Input: part model. Units: mm. Frame: model coordinates. Face numbers are marked on the shaded views. A direction names the side the tool comes from. Give positions to 0.01 mm unless a question says otherwise; leave off trailing zeros. Loops run counter-clockwise (first coordinate to the right, second up) from the corner with the lowest first, then second, coordinate; pieces in that order, holes last.
from build123d import *

# Parameters (mm, degrees)
F0_W     = 31.75
F0_H     = 82.55
F1_DEPTH = 6.35
F3_DEPTH = 6.35
F2_W     = 12.7
F2_H     = 29.119744
F4_DEPTH = 31.75
F6_DEPTH = 44.45
F8_DEPTH = 6.35


with BuildPart() as f1:
    # F0 (on Top) → F1 (new body)
    with BuildSketch(Plane.XY):
        with Locations((15.875, 0)):
            Rectangle(F0_W, F0_H)
    extrude(amount=F1_DEPTH)

    # F2 (on face) → F3 (join)
    with BuildSketch(Plane.YZ.offset(31.75)):
        Polygon((-41.275, 44.45), (-41.275, 6.35), (31.205256, 6.35), (-19.594744, 44.45), (-19.594744, 53.430256), (-32.294744, 53.430256), align=None)
        with BuildLine():
            ThreePointArc((-12.355744, 28.448), (-10.704744, 27.305), (-10.069744, 25.4))
            ThreePointArc((-10.069744, 25.4), (-10.704744, 23.495), (-12.355744, 22.352))
            ThreePointArc((-12.355744, 22.352), (-13.244744, 22.225), (-14.133744, 22.352))
            ThreePointArc((-14.133744, 22.352), (-16.419744, 25.4), (-14.133744, 28.448))
            ThreePointArc((-14.133744, 28.448), (-13.244744, 28.575), (-12.355744, 28.448))
        make_face(mode=Mode.SUBTRACT)
        with BuildLine():
            Line((-12.355744, 22.352), (-12.355744, 28.448))
            ThreePointArc((-12.355744, 28.448), (-13.244744, 28.575), (-14.133744, 28.448))
            Line((-14.133744, 28.448), (-14.133744, 22.352))
            ThreePointArc((-14.133744, 22.352), (-13.244744, 22.225), (-12.355744, 22.352))
        make_face()
    extrude(amount=-F3_DEPTH)

    # F2 (on face) → F4 (join)
    with BuildSketch(Plane.YZ.offset(31.75)):
        with Locations((-25.944744, 67.990128)):
            Rectangle(F2_W, F2_H)
    extrude(amount=-F4_DEPTH)

    # F5 (on face) → F6 (join)
    with BuildSketch(Plane.XZ.offset(41.275)):
        Polygon((25.4, 6.35), (0, 6.35), (0, 0), (31.75, 0), (31.75, 6.35), align=None)
    extrude(amount=F6_DEPTH)

    # F7 (on face) → F8 (join)
    with BuildSketch(Plane.YZ.offset(31.75)):
        Polygon((-41.275, 44.45), (-85.725, 6.35), (-79.375, 6.35), (-41.275, 39.007143), align=None)
    extrude(amount=-F8_DEPTH)

    # F9: F1 across plane


with BuildPart() as f1_1:
    add(f1.part)
    add(f1.part.mirror(Plane.YZ))


solid = f1_1.part
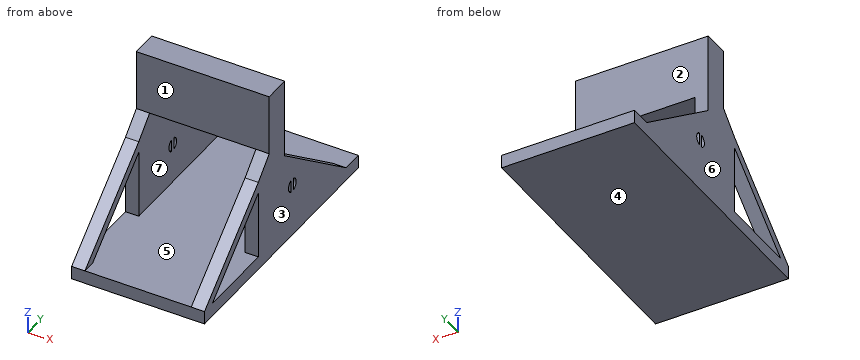
(1) Pin query (flat end, axial travel): pin 1 Ø3 at (x, z) = (29.5, 26) entering from +Y; pin 2 Ø5 at (x, z) = (-29.5, 31) entering from -Y; pin 3 Ø3 at (x, y) = (20.5, -16.5) entering from -Z; pin 4 Ø23.5 at (x, z) = (10, 69.5) entering from -Y. Return the tip coordinate at first contact, or that it passes through.
Values follow:
pin 1: stops at y = 7.01
pin 2: stops at y = -59.88
pin 3: stops at z = 0
pin 4: stops at y = -32.29
(2) Mould query, pull axis X, two halves, no side actions, for the marked faces 4, 5, 6 and 7. Classes: +X half, -X half, draft (parallel to the pull), parting line (faces both ways), or undercut.
Values follow:
face 4: draft
face 5: undercut
face 6: -X half
face 7: undercut
(3) Cut plane B-B (y = -24). Return the cut outline in (x, z), and give its area (3 significant figures).
Values follow:
outline: (-31.75, 0) - (31.75, 0) - (31.75, 82.55) - (-31.75, 82.55) - close; hole (-25.4, 6.35) - (25.4, 6.35) - (25.4, 53.43) - (-25.4, 53.43) - close
area: 2,850 mm2
(4) Cut plane C-C (z = 46). Return the cut outline in (x, y) (3 decimals).
Values follow:
outline: (-31.75, -39.725) - (-25.4, -39.725) - (-25.4, -19.595) - (-31.75, -19.595) - close; (25.4, -39.725) - (31.75, -39.725) - (31.75, -19.595) - (25.4, -19.595) - close
(5) Cut plane D-D (z = 30). Return the cut outline in (x, y) (3 decimals).
Values follow:
outline: (-31.75, -58.133) - (-25.4, -58.133) - (-25.4, -51.783) - (-31.75, -51.783) - close; (-31.75, -41.275) - (-25.4, -41.275) - (-25.4, -0.328) - (-31.75, -0.328) - close; (25.4, -58.133) - (31.75, -58.133) - (31.75, -51.783) - (25.4, -51.783) - close; (25.4, -41.275) - (31.75, -41.275) - (31.75, -0.328) - (25.4, -0.328) - close
(6) Ray query, probe 1 along X at (y, z) = (-15, 21); probe 2 along Y at (x, z) = (24, 65); probe 3 along Z at (x, y) = (12, -23). Return the intervals inside material, ascending.
Values follow:
probe 1: x = -31.75 to -25.4, 25.4 to 31.75
probe 2: y = -32.29 to -19.59
probe 3: z = 0 to 6.35, 53.43 to 82.55
(7) Cut plane A-A (x = -3). Return the cut outline in (y, z) (3 decimals).
Values follow:
outline: (-85.725, 0) - (41.275, 0) - (41.275, 6.35) - (-85.725, 6.35) - close; (-32.295, 53.43) - (-19.595, 53.43) - (-19.595, 82.55) - (-32.295, 82.55) - close
(8) Reachability of the marked faces 1, 2 and 3 from +Z, -Z, +X, -X, +Y, -Y: full face, straight path, thin tool, end or side. Return the list, or none.
Values follow:
face 1: +Z, +X, -X, -Y
face 2: +Z, +X, -X, +Y
face 3: +Z, -Z, +X, +Y, -Y
